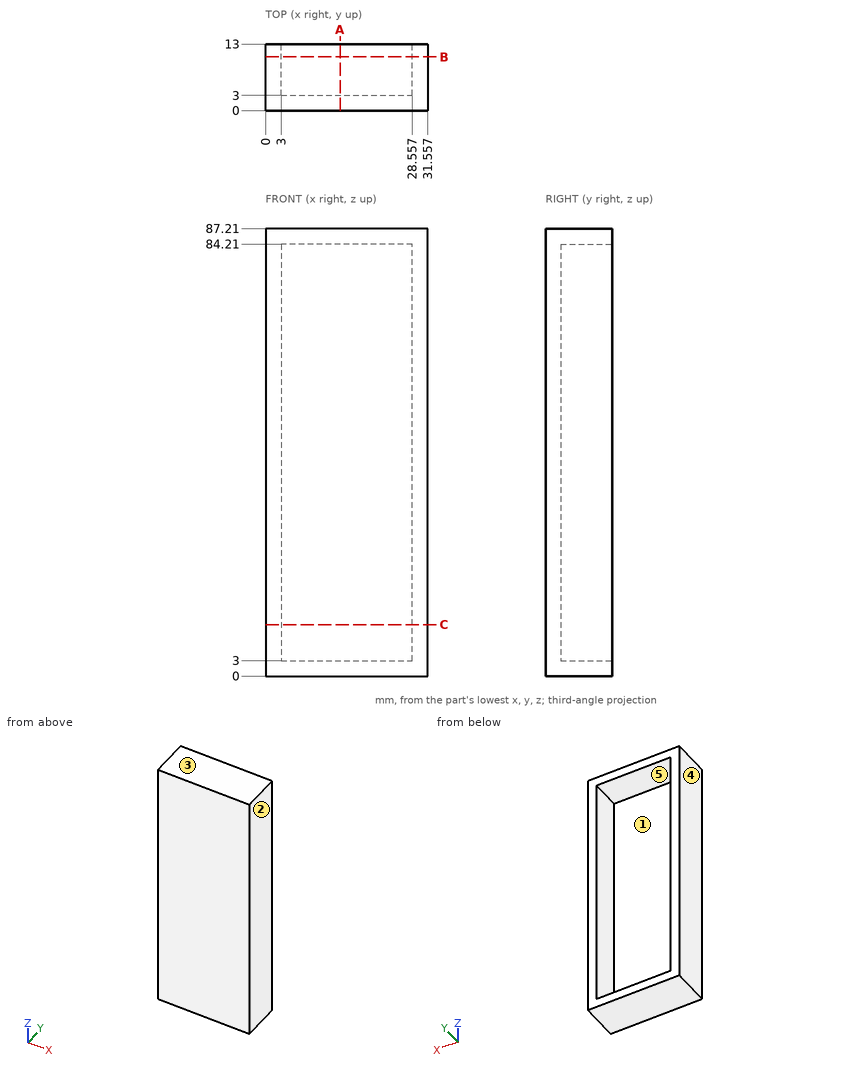
Print and shaded views of the part. All mm, measured from the part's lowest x, y and z. A direction names the side the tool comes from. Round coordinates to 2 decimals unless told otherwise and drop trailing zeros. Order: outer loops, then holes, each group sorted by start corner. A loop starts at its lowest first (then second) coordinate and runs counter-clockwise, first axis right, second up. Notation, with made-up numbers: (14.25, -16.5) - (30.25, -16.5) arc R20 cw to (30.25, -12.5) - close; hole circle Ø11 at (-27.5, -16). An arc over 180 degrees is marked (long way). Use a Markdown table: item, result.
1) Saw through at A-A on x = 14.5. Write the cut outline in (y, z).
Recorded:
| item | result |
|---|---|
| outline | (0, 0) - (13, 0) - (13, 3) - (3, 3) - (3, 84.21) - (13, 84.21) - (13, 87.21) - (0, 87.21) - close |
2) Saw through at C-C on z = 10. Write the cut outline in (x, y), and give its area (3 significant figures).
Recorded:
| item | result |
|---|---|
| outline | (0, 0) - (31.56, 0) - (31.56, 13) - (28.56, 13) - (28.56, 3) - (3, 3) - (3, 13) - (0, 13) - close |
| area | 155 mm² |
3) Wall check: L1, parallel to X at y = 5, z = 46; L2, parallel to Z at x = 16, y = 3.5; L3, parallel to Y at x = 24, z = 68.5. Give the ranges that are in metal, low to high.
Recorded:
| item | result |
|---|---|
| L1 | x = 0 to 3, 28.56 to 31.56 |
| L2 | z = 0 to 3, 84.21 to 87.21 |
| L3 | y = 0 to 3 |
4) Pull direction X, two halves, no side cores. Call the marked faces 1, 2 and 3: pulls with the +X half, pulls with the -X half, needs draft (parallel to the pull), parting line crosses it, or undercut.
Recorded:
| item | result |
|---|---|
| face 1 | undercut |
| face 2 | pulls with the +X half |
| face 3 | needs draft |
5) Saw through at B-B on y = 10.5. Write the cut outline in (x, z).
Recorded:
| item | result |
|---|---|
| outline | (0, 0) - (31.56, 0) - (31.56, 87.21) - (0, 87.21) - close; hole (3, 3) - (28.56, 3) - (28.56, 84.21) - (3, 84.21) - close |
6) Tool access for the marked faces 4 and 5: list every direction of +Z, -Z, +X, -X, +Y, -Y with a clear straight run to the whole face (end or side of a thin tool).
Recorded:
| item | result |
|---|---|
| face 4 | +Z, -Z, -X, +Y, -Y |
| face 5 | +Y |
7) Flat gauge pin, fed straight in: pin 1 Ø13 at (x, z) = (10.5, 42.5) entering from +Y. Where does the tip first touch, or does it go through?
Recorded:
| item | result |
|---|---|
| pin 1 | stops at y = 3 |
